Design review of the part built by this model. Coordinates are the model's own, in mm. Coordinates: 2 decimals unless noted, no trailing zeros. Loops run counter-clockwise (first coordinate to the right, second up) from the corner with the lowest first, then second, coordinate; pieces in that order, holes last. Notation, with made-up numbers: M -32,61.5 L 11,61.5 A25 cw 11,90.5 Z; hole C 30.5,-19 d7. An arc over 180 degrees is marked long. Answer as a JSON object with one key per item and string values. Group by question number.
1. To check wall thickness, follow probe 1 along X at (y, z) = (28, -1.5); probe 2 along X at (y, z) = (35, -2.5); probe 3 along Y at (x, z) = (197.5, -0.7). State the ranges of each line that lie inside material, in increasing order.
2. Consider section B-B (z = -0.8). State the section outline as (x, y) points.
3. Consider section A-A (y = 7). State the section outline as (x, z) points (3 decimals), then the cut area to 3 significant figures.
Autodesk Inventor part; units mm, degrees
ref_plane "YZ Plane" through (0, 0, 0) normal (1, 0, 0) x (0, 1, 0)
ref_plane "XZ Plane" through (0, 0, 0) normal (0, 1, 0) x (-1, 0, 0)
ref_plane "XY Plane" through (0, 0, 0) normal (0, 0, 1) x (1, 0, 0)
sketch "Sketch1" plane through (0, 0, 0) normal (0, 0, 1) x (1, 0, 0)
  line L0 (-228.6, 38.1) -> (190.5, 38.1)
  line L1 (228.6, 0) -> (228.6, -38.1)
  line L2 (228.6, -38.1) -> (-228.6, -38.1)
  line L3 (-228.6, -38.1) -> (-228.6, 38.1)
  line L4 (190.5, 38.1) -> (228.6, 0)
  point P0 (0, 0)
  dimension "d1" = 76.2
  dimension "d2" = 38.1
  dimension "d3" = 228.6
  dimension "d6" = 38.1
  dimension "d7" = 45
  dimension "d8" = 457.2
extrude "Extrusion1" add sketch "Sketch1" against normal blind 3.175
properties part number "Side_Panel"
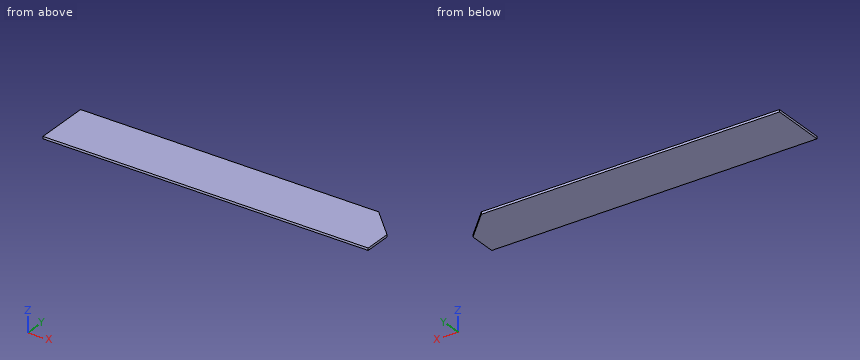
Findings below:
{
 "1": {"probe 1": "x = -228.6 to 200.6", "probe 2": "x = -228.6 to 193.6", "probe 3": "y = -38.1 to 31.1"},
 "2": {"outline": "M -228.6,-38.1 L 228.6,-38.1 L 228.6,0 L 190.5,38.1 L -228.6,38.1 Z"},
 "3": {"outline": "M -228.6,-3.175 L 221.6,-3.175 L 221.6,0 L -228.6,0 Z", "area": "1,430 mm^2"}
}
